from build123d import *

# Parameters (mm, degrees)
SKETCH1_W           = 140
SKETCH1_H           = 60
SKETCH1_R           = 7.5
SKETCH1_R_2         = 2.5
BOSS_EXTRUDE1_DEPTH = 3.2
CHAMFER1_SIZE       = 10


with BuildPart() as part:
    # Sketch1 → Boss-Extrude1 (new body)
    with BuildSketch(Plane.XY):
        Rectangle(SKETCH1_W, SKETCH1_H)
        Circle(SKETCH1_R, mode=Mode.SUBTRACT)
        with Locations((-10.5, 10.5)):
            Circle(SKETCH1_R_2, mode=Mode.SUBTRACT)
        with Locations((10.5, 10.5)):
            Circle(SKETCH1_R_2, mode=Mode.SUBTRACT)
        with Locations((10.5, -10.5)):
            Circle(SKETCH1_R_2, mode=Mode.SUBTRACT)
        with Locations((-10.5, -10.5)):
            Circle(SKETCH1_R_2, mode=Mode.SUBTRACT)
        with BuildLine():
            Line((-65.5, -11.5), (-65.5, 11.5))
            ThreePointArc((-65.5, 11.5), (-62, 15), (-58.5, 11.5))
            Line((-58.5, 11.5), (-58.5, -11.5))
            ThreePointArc((-58.5, -11.5), (-62, -15), (-65.5, -11.5))
        make_face(mode=Mode.SUBTRACT)
        with BuildLine():
            Line((58.5, -11.5), (58.5, 11.5))
            ThreePointArc((58.5, 11.5), (62, 15), (65.5, 11.5))
            Line((65.5, 11.5), (65.5, -11.5))
            ThreePointArc((65.5, -11.5), (62, -15), (58.5, -11.5))
        make_face(mode=Mode.SUBTRACT)
    extrude(amount=BOSS_EXTRUDE1_DEPTH)

    # Chamfer1
    chamfer1_edges = [part.edges().sort_by_distance(p)[0] for p in [
        (70, -30, 1.6),
        (-70, -30, 1.6),
        (-70, 30, 1.6),
        (70, 30, 1.6),
    ]]
    chamfer(chamfer1_edges, length=CHAMFER1_SIZE)


solid = part.part
The model under review builds one solid part; all positions refer to its coordinate system, in mm. A direction names the side the tool comes from. Give positions to 0.01 mm unless a question says otherwise; leave off trailing zeros. Write each loop counter-clockwise with the first axis right and the second up, starting at its lowest first coordinate (ties: lowest second). Pieces come first, ordered by that corner, then holes.
1. Wall thickness on L1, parallel to X at y = -0.5, z = 0.7; L2, parallel to X at y = 5.5, z = 1.15; L3, parallel to Y at x = 9.5, z = 1.9: over which ranges is each line inside the solid? List them lowest first.
2. Add section C-C, the plane x = -62. Write out the cut boundary in (y, z), plus the area to 3 significant figures.
3. Add section D-D, the plane z = 2.5. Write out the cut boundary in (x, y), plus the area to 3 significant figures.
4. Add section A-A, the plane x = -10.5. Write out the cut boundary in (y, z).
5. Add section B-B, the plane y = 0. Write out the cut boundary in (x, z).
6. Draft analysis for pull direction Y (two halves, no side actions). For faces 1 (the cylindrical face through (-11.04, 8.06, 1.58)), 2 (the flat face through (-65, -25, 2)), 3 (the flat face through (70, 0, 2)), 4 (the flat face through (65, 25, 2)), state which applies: +Y half, -Y half, draft (parallel to the pull), parting line (faces both ways), or undercut.
7. Tool access review of faces 5 (the flat face through (-1, 30, 2)), 6 (the cylindrical face through (-62, 15, 2)): name each direction out of +Z, -Z, +X, -X, +Y, -Y from which nothing blocks a thin tool from reaching the whole face with its end or side.
Worked answers:
1. L1: x = -70 to -65.5, -58.5 to -7.48, 7.48 to 58.5, 65.5 to 70
1. L2: x = -70 to -65.5, -58.5 to -5.1, 5.1 to 58.5, 65.5 to 70
1. L3: y = -30 to -12.79, -8.21 to 8.21, 12.79 to 30
2. outline: (-28, 0) - (-15, 0) - (-15, 3.2) - (-28, 3.2) - close; (15, 0) - (28, 0) - (28, 3.2) - (15, 3.2) - close
2. area: 83.2 mm2
3. outline: (-70, -20) - (-60, -30) - (60, -30) - (70, -20) - (70, 20) - (60, 30) - (-60, 30) - (-70, 20) - close; hole (-65.5, -11.5) arc R3.5 ccw to (-58.5, -11.5) - (-58.5, 11.5) arc R3.5 ccw to (-65.5, 11.5) - close; hole circle Ø5 at (-10.5, -10.5); hole circle Ø5 at (-10.5, 10.5); hole circle Ø15 at (0, 0); hole circle Ø5 at (10.5, -10.5); hole circle Ø5 at (10.5, 10.5); hole (58.5, -11.5) arc R3.5 ccw to (65.5, -11.5) - (65.5, 11.5) arc R3.5 ccw to (58.5, 11.5) - close
3. area: 7,550 mm2
4. outline: (-30, 0) - (-13, 0) - (-13, 3.2) - (-30, 3.2) - close; (-8, 0) - (8, 0) - (8, 3.2) - (-8, 3.2) - close; (13, 0) - (30, 0) - (30, 3.2) - (13, 3.2) - close
5. outline: (-70, 0) - (-65.5, 0) - (-65.5, 3.2) - (-70, 3.2) - close; (-58.5, 0) - (-7.5, 0) - (-7.5, 3.2) - (-58.5, 3.2) - close; (7.5, 0) - (58.5, 0) - (58.5, 3.2) - (7.5, 3.2) - close; (65.5, 0) - (70, 0) - (70, 3.2) - (65.5, 3.2) - close
6. face 1: undercut
6. face 2: -Y half
6. face 3: draft
6. face 4: +Y half
7. face 5: +Z, -Z, +X, -X, +Y
7. face 6: +Z, -Z
